```python
from build123d import *

# Parameters (mm, degrees)
SKETCH1_R                = 5
SKETCH1_R_2              = 2.5
BOSS_EXTRUDE1_DEPTH      = 3
BOSS_EXTRUDE1_DEPTH_BACK = 2
SKETCH2_R                = 5
BOSS_EXTRUDE2_DEPTH      = 1
SKETCH3_R                = 1.15
CUT_EXTRUDE1_DEPTH       = 1


with BuildPart() as part:
    # Sketch1 → Boss-Extrude1 (new body, two sides)
    with BuildSketch(Plane(origin=(0, 0, 0), x_dir=(1, 0, 0), z_dir=(0, 1, 0))) as boss_extrude1_sk:
        Circle(SKETCH1_R)
        Circle(SKETCH1_R_2, mode=Mode.SUBTRACT)
    extrude(amount=BOSS_EXTRUDE1_DEPTH)
    extrude(boss_extrude1_sk.sketch, amount=-BOSS_EXTRUDE1_DEPTH_BACK)

    # Sketch2 → Boss-Extrude2 (add)
    with BuildSketch(Plane.XZ.offset(2)):
        Circle(SKETCH2_R)
    extrude(amount=BOSS_EXTRUDE2_DEPTH)

    # Sketch3 → Cut-Extrude1 (cut)
    with BuildSketch(Plane.XZ.offset(3)):
        Circle(SKETCH3_R)
    extrude(amount=-CUT_EXTRUDE1_DEPTH, mode=Mode.SUBTRACT)


solid = part.part
```
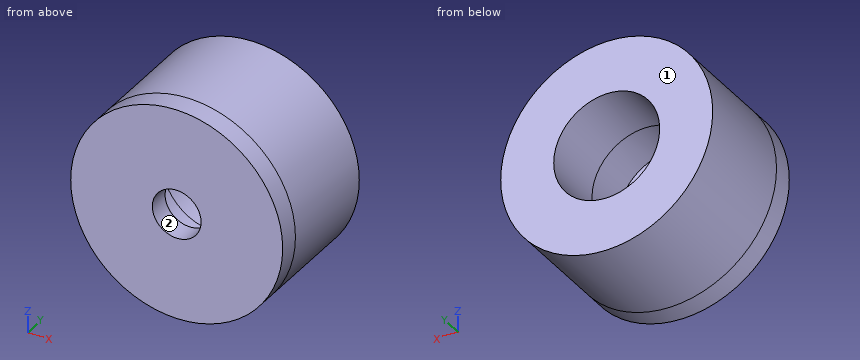
Work out the finished part from the listing and answer in its coordinate system (mm). Face numbers are marked on the shaded views. Coordinates: 2 decimals unless noted, no trailing zeros. Write each loop counter-clockwise with the first axis right and the second up, starting at its lowest first coordinate (ties: lowest second). Pieces come first, ordered by that corner, then holes. Notation, with made-up numbers: (60, -8) - (71, -8) arc R14 cw to (71, 10) - close; hole circle Ø6 at (-25, -8). An arc over 180 degrees is marked (long way). Answer as a JSON object with one key per item and string values.
Q1. Find section A-A (z = 0). Write down the section's boundary in (x, y), plus the area to 3 significant figures.
Results list:
{"outline": "(-5, -3) - (-1.15, -3) - (-1.15, -2) - (-2.5, -2) - (-2.5, 3) - (-5, 3) - close; (1.15, -3) - (5, -3) - (5, 3) - (2.5, 3) - (2.5, -2) - (1.15, -2) - close", "area": "32.7 mm^2"}
Q2. Consider L1, parallel to X at y = 1.7, z = 0; L2, parallel to Z at x = 0, y = -2.4. Determine where each line is inside the solid, lowest interval first. Write a range as from..to.
Results list:
{"L1": "x = -5..-2.5, 2.5..5", "L2": "z = -5..-1.15, 1.15..5"}
Q3. Find section B-B (x = 0). Write down the section's boundary in (y, z), plus the area to 3 significant figures.
Results list:
{"outline": "(-3, -5) - (3, -5) - (3, -2.5) - (-2, -2.5) - (-2, -1.15) - (-3, -1.15) - close; (-3, 1.15) - (-2, 1.15) - (-2, 2.5) - (3, 2.5) - (3, 5) - (-3, 5) - close", "area": "32.7 mm^2"}
Q4. Find section D-D (z = 2.25). Write down the section's boundary in (x, y), plus the area to 3 significant figures.
Results list:
{"outline": "(-4.47, -3) - (4.47, -3) - (4.47, 3) - (1.09, 3) - (1.09, -2) - (-1.09, -2) - (-1.09, 3) - (-4.47, 3) - close", "area": "42.7 mm^2"}
Q5. Find section C-C (y = 2.05). Write down the section's boundary in (x, z).
Results list:
{"outline": "circle Ø10 at (0, 0); hole circle Ø5 at (0, 0)"}
Q6. Given pin 1 Ø3 at (x, z) = (0, 0) entering from +Y; pin 2 Ø2 at (x, z) = (0, 0) entering from -Y; pin 3 Ø2 at (x, y) = (2, -1) entering from +Z, each flat-ended and moving along its own axis, determine where each tip first touches the part or whether it passes through.
Results list:
{"pin 1": "stops at y = -2", "pin 2": "passes through", "pin 3": "stops at z = 4.9"}
Q7. For a pull along Z with two mould halves and no side action, classify the marked faces 1 and 2 as pulls with the +Z half, pulls with the -Z half, needs draft (parallel to the pull), parting line crosses it, or undercut.
Results list:
{"face 1": "needs draft", "face 2": "undercut"}
